The model under review builds one solid part; all positions refer to its coordinate system, in mm. Coordinates: 2 decimals unless noted, no trailing zeros. Put each result on its own line as item: value. Start each with the question number.
Item 1: For pin 1 (1.9 mm diameter, centred on x = 73.29, y = -7.34, fed in from -Z); pin 2 (4 mm diameter, centred on x = 70.79, y = 12.11, fed in from +Z), all flat-tipped, find the tip position at first contact; note any pin that passes through.
Item 2: Consider section A-A on z = -4.55. State how many separate pieces and enclosed holes the cut face has, then the cut area to 3 significant figures.
Item 3: To check wall thickness, follow L1, parallel to Y at x = 92.25, z = -3.1; L2, parallel to X at y = 8, z = -4.85; L3, parallel to Y at x = 93, z = -4.1. State the ranges of each line that lie inside material, in increasing order. Write a range as [from, to].
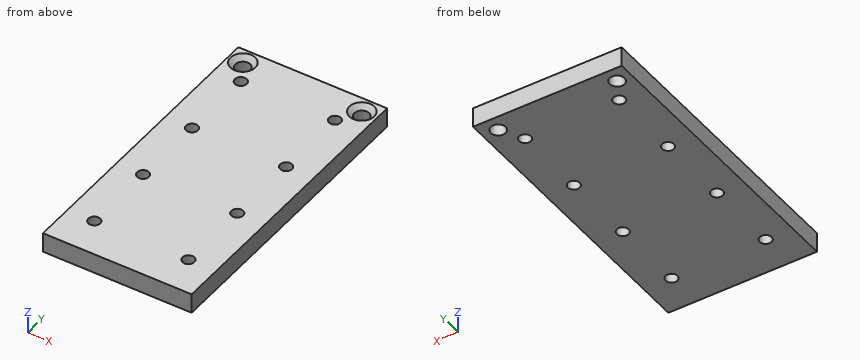
Autodesk Inventor part; units mm, degrees
ref_plane "YZ Plane" through (0, 0, 0) normal (1, 0, 0) x (0, 1, 0)
ref_plane "XZ Plane" through (0, 0, 0) normal (0, 1, 0) x (-1, 0, 0)
ref_plane "XY Plane" through (0, 0, 0) normal (0, 0, 1) x (1, 0, 0)
ref_plane "РабПлоскость2" through (101.7859, 42.6575, -2.4) normal (0, 0, -1) x (-1, 0, 0)
sketch "Эскиз2" plane through (101.7859, 42.6575, -2.4) normal (0, 0, -1) x (-1, 0, 0)
  line L0 (6.2, -87.5) -> (12.8, -87.5)
  line L1 (12.8, -7.5) -> (12.8, -87.5)
  line L2 (6.2, -7.5) -> (6.2, -87.5)
  circle A0 centre (9.5, -35) radius 2.3
  circle A1 centre (9.5, -50) radius 2.3
  circle A2 centre (9.5, -65) radius 2.3
  circle A3 centre (9.5, -80) radius 2.3
  line L3 (25.2, -87.5) -> (31.8, -87.5)
  line L4 (31.8, -7.5) -> (31.8, -87.5)
  line L5 (25.2, -7.5) -> (25.2, -87.5)
  circle A4 centre (28.5, -35) radius 2.3
  circle A5 centre (28.5, -50) radius 2.3
  circle A6 centre (28.5, -65) radius 2.3
  circle A7 centre (28.5, -80) radius 2.3
  line L6 (3.9216, -27.5) -> (33.9216, -27.5)
  line L7 (33.9216, -27.5) -> (33.9216, -87.5)
  line L8 (33.9216, -87.5) -> (3.9216, -87.5)
  line L9 (3.9216, -87.5) -> (3.9216, -27.5)
  line L10 (18.9216, -50) -> (18.9216, -69.7785)
  circle A8 centre (9.5, -35) radius 1.2
  circle A9 centre (9.5, -50) radius 1.2
  circle A10 centre (9.5, -65) radius 1.2
  circle A11 centre (9.5, -80) radius 1.2
  circle A12 centre (28.5, -80) radius 1.2
  circle A13 centre (28.5, -65) radius 1.2
  circle A14 centre (28.5, -50) radius 1.2
  circle A15 centre (28.5, -35) radius 2.1
  circle A16 centre (28.5, -35) radius 1.2
  line L11 (25.2, -7.5) -> (31.8, -7.5)
  line L12 (6.2, -7.5) -> (12.8, -7.5)
  point P0 (101.7859, -42.6575)
  dimension "d3" = 30
  dimension "d4" = 60
  dimension "d5" = 15
extrude "Выдавливание2" add sketch "Эскиз2" along normal blind 4 contours L2 L6 L1 L0 | L8 L9 L6 L2 | L1 L6 L5 L8 | L5 L6 L4 L3 | L4 L6 L7 L8 | A0 | A1 | A2 | A3 | A4 | A5 | A6 | A7 | A15
sketch "Эскиз3" plane through (101.7859, 42.6575, -6.4) normal (0, 0, -1) x (-1, 0, 0)
  circle A0 centre (7, -34.5989) radius 2
  circle A1 centre (31, -34.5989) radius 2
  circle A2 centre (7, -30.55) radius 1.5
  circle A3 centre (31, -30.55) radius 1.5
  circle A4 centre (7, -30.55) radius 1.5
  point P0 (101.7859, -42.6575)
extrude "Выдавливание3" cut sketch "Эскиз3" against normal blind 10 contours A2 | A3
chamfer "Фаска1" distance 1 angle 45 2 edges at (96.2859, 12.1075, -2.4) (72.2859, 12.1075, -2.4)
properties part number "деталь которая двигает"
Report:
1. pin 1: through
1. pin 2: z = -2.9
2. separate pieces: 1
2. enclosed holes: 10
2. area: 1,750 mm²
3. L1: [-44.84, -38.54], [-36.14, -23.54], [-21.14, -8.54], [-6.14, 6.46], [8.86, 15.16]
3. L2: [67.86, 72.14], [74.44, 91.14], [93.44, 97.86]
3. L3: [-44.84, -38.31], [-36.38, -23.31], [-21.38, -8.31], [-6.38, 6.69], [8.62, 15.16]
